Model file for the job. Use its own axes, mm. Face numbers are marked on the shaded views. A direction names the side the tool comes from. Coordinates: 2 decimals unless noted, no trailing zeros. Loops run counter-clockwise (first coordinate to the right, second up) from the corner with the lowest first, then second, coordinate; pieces in that order, holes last.
Autodesk Fusion 360 part; units mm, degrees
sketch "Sketch1" plane through (0, 0, 0) normal (0, 1, 0) x (1, 0, 0)
  line L0 (41.5, 41.5) -> (-41.5, 41.5)
  line L1 (-41.5, -41.5) -> (41.5, -41.5)
  line L2 (-41.5, 41.5) -> (41.5, -41.5) construction
  line L3 (41.5, 41.5) -> (41.5, 17)
  line L4 (41.5, 17) -> (34.5, 17)
  line L5 (-41.5, 41.5) -> (-41.5, 17)
  line L6 (-41.5, 17) -> (-34.5, 17)
  line L7 (-41.5, -17) -> (-34.5, -17)
  line L8 (41.5, -17) -> (34.5, -17)
  line L9 (-34.5, 17) -> (-34.5, -17)
  line L10 (34.5, 17) -> (34.5, -17)
  line L11 (-41.5, 41.5) -> (-41.5, 17)
  line L12 (-41.5, -17) -> (-41.5, -41.5)
  line L13 (-41.5, -41.5) -> (-41.5, -17)
  line L14 (-41.5, 17) -> (-41.5, 41.5)
  line L15 (41.5, -41.5) -> (41.5, -17)
  line L16 (41.5, 17) -> (41.5, 41.5)
  line L17 (41.5, 41.5) -> (41.5, 17)
  line L18 (41.5, -17) -> (41.5, -41.5)
  line L19 (-34.5, 17) -> (-34.5, 8.6)
  line L20 (-34.5, -17) -> (-34.5, -8.6)
  line L21 (34.5, 17) -> (34.5, 8.6)
  line L22 (34.5, -17) -> (34.5, -8.6)
  line L23 (-41.5, 41.5) -> (-33.655, 41.5)
  line L24 (-33.655, 41.5) -> (-41.5, 41.5)
  line L25 (-41.5, 41.5) -> (-41.5, 33.655)
  circle A0 centre (-33.655, 33.655) radius 1.55
  circle A1 centre (33.655, 33.655) radius 1.55
  circle A2 centre (-33.655, -33.655) radius 1.55
  circle A3 centre (33.655, -33.655) radius 1.55
  line L26 (11, 11) -> (-11, -11) construction
  line L27 (-11, 11) -> (11, -11) construction
  line L28 (12.5, -12.5) -> (-12.5, -12.5)
  line L29 (-12.5, -12.5) -> (-12.5, 12.5)
  line L30 (-12.5, 12.5) -> (12.5, 12.5)
  line L31 (12.5, 12.5) -> (12.5, -12.5)
  line L32 (12.5, -12.5) -> (-12.5, 12.5) construction
  line L33 (-12.5, -12.5) -> (12.5, 12.5) construction
  line L34 (-41.5, 41.5) -> (-14.05, 41.5)
  line L35 (-14.05, 41.5) -> (-8.5, 41.5)
  circle A4 centre (-8.5, 33.655) radius 1.55
  circle A5 centre (8.5, 33.655) radius 1.55
  line L36 (-14.05, 41.5) -> (-14.05, 23.5)
  line L37 (-14.05, 23.5) -> (14.05, 23.5)
  line L38 (14.05, 23.5) -> (14.05, 41.5)
  line L39 (-14.05, -23.5) -> (14.05, -23.5)
  circle A6 centre (8.5, -33.655) radius 1.55
  circle A7 centre (-8.5, -33.655) radius 1.55
  line L40 (-14.05, -41.5) -> (-14.05, -23.5)
  line L41 (14.05, -23.5) -> (14.05, -41.5)
  circle A8 centre (-19.5, 8.6) radius 1.55
  circle A9 centre (-19.5, -8.6) radius 1.55
  circle A10 centre (19.5, 8.6) radius 1.55
  circle A11 centre (19.5, -8.6) radius 1.55
  point P0 (-19.5, 8.6)
  point P1 (19.5, 8.6)
  dimension "d1" = 83
  dimension "d2" = 83
  dimension "d31" = 27.45
  dimension "d32" = 5.55
  dimension "d33" = 7.845
  dimension "d34" = 17
  dimension "d35" = 3.1
  dimension "d36" = 3.1
  dimension "d37" = 18
  dimension "d39" = 18
  dimension "d40" = 3.1
extrude "Extrude4" add sketch "Sketch1" along normal blind 8 contours L0 L1 L3 L4 L5 L6 L7 L8 L9 L10 L11 L12 L13 L14 L15 L16 L17 L18 L19 L20 L21 L22 L23 L24 L25 L34 L36 L37 L38 L39 L40 L41 makes body 1
sketch "Sketch2" plane through (0, 8, 0) normal (0, 1, 0) x (-1, 0, 0)
  circle A0 centre (-19.5, -8.6) radius 1.55
  circle A1 centre (33.655, 33.655) radius 1.55
  circle A2 centre (19.5, -8.6) radius 1.55
  circle A3 centre (19.5, 8.6) radius 1.55
  circle A4 centre (-19.5, 8.6) radius 1.55
  line L0 (12.5, -12.5) -> (-12.5, -12.5)
  line L1 (-12.5, -12.5) -> (-12.5, 12.5)
  line L2 (-12.5, 12.5) -> (12.5, 12.5)
  line L3 (12.5, 12.5) -> (12.5, -12.5)
  circle A5 centre (-33.655, -33.655) radius 1.55
  circle A6 centre (33.655, -33.655) radius 1.55
  circle A7 centre (-33.655, 33.655) radius 1.55
  line L4 (41.5, 41.5) -> (14.05, 41.5)
  line L5 (14.05, 41.5) -> (14.05, 23.5)
  line L6 (14.05, 23.5) -> (-14.05, 23.5)
  line L7 (-14.05, 23.5) -> (-14.05, 41.5)
  line L8 (-14.05, 41.5) -> (-41.5, 41.5)
  line L9 (-41.5, 41.5) -> (-41.5, 17)
  line L10 (-41.5, 17) -> (-34.5, 17)
  line L11 (-34.5, 17) -> (-34.5, -17)
  line L12 (-34.5, -17) -> (-41.5, -17)
  line L13 (-41.5, -17) -> (-41.5, -41.5)
  line L14 (-41.5, -41.5) -> (-14.05, -41.5)
  line L15 (-14.05, -41.5) -> (-14.05, -23.5)
  line L16 (-14.05, -23.5) -> (14.05, -23.5)
  line L17 (14.05, -23.5) -> (14.05, -41.5)
  line L18 (14.05, -41.5) -> (41.5, -41.5)
  line L19 (41.5, -41.5) -> (41.5, -17)
  line L20 (41.5, -17) -> (34.5, -17)
  line L21 (34.5, -17) -> (34.5, 17)
  line L22 (34.5, 17) -> (41.5, 17)
  line L23 (41.5, 17) -> (41.5, 41.5)
extrude "Extrude5" cut sketch "Sketch2" against normal blind 3 keep common part bodies 1
sketch "Sketch3" plane through (0, 0, 23.5) normal (0, 0, 1) x (1, 0, 0)
  line L0 (-14.05, 5) -> (14.05, 5)
  line L1 (14.05, 5) -> (14.05, 8)
  line L2 (14.05, 8) -> (-14.05, 8)
  line L3 (-14.05, 8) -> (-14.05, 5)
  line L4 (-14.05, 8) -> (-14.05, 0)
  line L5 (-14.05, 0) -> (14.05, 0)
  line L6 (14.05, 0) -> (14.05, 8)
  line L7 (14.05, 8) -> (-14.05, 8)
  line L8 (-14.05, 8) -> (-14.05, 0)
  line L9 (-14.05, 0) -> (14.05, 0)
  dimension "d47" = 28.1
extrude "Extrude6" add sketch "Sketch3" against normal blind 3 contours L0 L4 L5 L6 L8 L9 bodies 1
extrude "Extrude7" add sketch "Sketch1" against normal blind 3 separate body contours L1 L39 L40 L41 makes body 2
sketch "Sketch4" plane through (0, 0, 23.5) normal (0, 0, 1) x (1, 0, 0)
  line L0 (14.05, 5) -> (14.05, 8)
  line L1 (14.05, 8) -> (-14.05, 8)
  line L2 (-14.05, 8) -> (-14.05, 5)
  line L3 (-14.05, 5) -> (-14.05, 0)
  line L4 (-14.05, 0) -> (14.05, 0)
  line L5 (14.05, 0) -> (14.05, 5)
  line L6 (-14.05, 0) -> (-14.05, -3)
  line L7 (-14.05, -3) -> (14.05, -3)
  line L8 (-14.05, 0) -> (14.05, 0)
  line L9 (14.05, 0) -> (14.05, -3)
  line L10 (14.05, -3) -> (-14.05, -3)
  line L11 (-14.05, -3) -> (-14.05, 0)
  dimension "d52" = 3
  dimension "d53" = 28.1
extrude "Extrude8" add sketch "Sketch4" against normal blind 3 contours L4 L6 L7 L8 L9 L10 L11 bodies 1 2
sketch "Sketch5" plane through (0, 0, -23.5) normal (0, 0, -1) x (-1, 0, 0)
  line L0 (-14.05, 5) -> (14.05, 5)
  line L1 (14.05, 5) -> (14.05, 8)
  line L2 (14.05, 8) -> (-14.05, 8)
  line L3 (-14.05, 8) -> (-14.05, 5)
  line L4 (-14.05, 5) -> (-14.05, -3)
  line L5 (-14.05, -3) -> (14.05, -3)
  line L6 (14.05, -3) -> (-14.05, -3)
  line L7 (-14.05, -3) -> (-14.05, 5)
  line L8 (-14.05, 5) -> (14.05, 5)
  line L9 (14.05, 5) -> (14.05, -3)
  dimension "d56" = 8
  dimension "d57" = 28.1
extrude "Extrude9" add sketch "Sketch5" against normal blind 3 contours L0 L4 L5 L6 L7 L8 L9 bodies 1
extrude "Extrude10" add sketch "Sketch1" against normal blind 3 contours L0 L35 L36 L37 L38 bodies 1
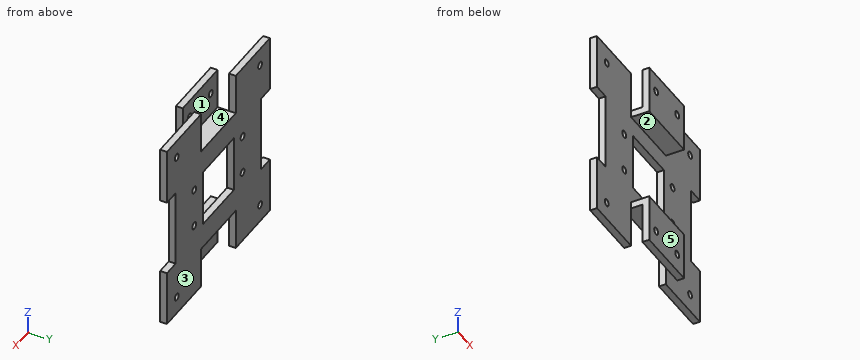
Q1. Slice it at A-A (x = -3). List the corners of the cut face in (y, z).
Answers:
outline: (-3, -41.5) - (0, -41.5) - (0, -23.5) - (8, -23.5) - (8, -12.5) - (5, -12.5) - (5, -20.5) - (-3, -20.5) - close; (-3, 20.5) - (5, 20.5) - (5, 12.5) - (8, 12.5) - (8, 23.5) - (0, 23.5) - (0, 41.5) - (-3, 41.5) - close
Q2. Which spindle directions (+Z, -Z, +X, -X, +Y, -Y) get a long thin tool onto all of the face, cutting with end or side? Do the marked faces 1, 2 and 3. Say none if no direction does.
Answers:
face 1: +Z, +X, -X, +Y
face 2: +X, -X, -Y
face 3: +Z, -Z, +X, -X, +Y
Q3. Slice it at D-D (z = -8.6). List the corners of the cut face in (x, y).
Answers:
outline: (-34.5, 5) - (-21.05, 5) - (-21.05, 8) - (-34.5, 8) - close; (-17.95, 5) - (-12.5, 5) - (-12.5, 8) - (-17.95, 8) - close; (12.5, 5) - (17.95, 5) - (17.95, 8) - (12.5, 8) - close; (21.05, 5) - (34.5, 5) - (34.5, 8) - (21.05, 8) - close
Q4. Slice it at B-B (y = -1.25). List the corners of the cut face in (x, z) (3 decimals).
Answers:
outline: (-14.05, -41.5) - (14.05, -41.5) - (14.05, -20.5) - (-14.05, -20.5) - close; (-14.05, 20.5) - (14.05, 20.5) - (14.05, 41.5) - (-14.05, 41.5) - close; hole circle Ø3.1 at (-8.5, -33.655); hole circle Ø3.1 at (-8.5, 33.655); hole circle Ø3.1 at (8.5, -33.655); hole circle Ø3.1 at (8.5, 33.655)
Q5. Flat gauge pins, fed straight in: P1, Ø0.9, axis at x = -3.5, y = 7, coming from the -Z side; P2, Ø3, axis at x = -8.5, z = 33.655, coming from the +Y side; P3, Ø3.5, axis at y = 6.5, z = -4.5, coming from the -X side; P4, Ø1.5, axis at y = 7, z = 1.5, coming from the +X side. Where does each tip first touch, or does it go through?
Answers:
P1: stops at z = -23.5
P2: passes through
P3: stops at x = -34.5
P4: stops at x = 34.5
Q6. Mould opens along X. For the marked faces 4 and 5 say: +X half, -X half, draft (parallel to the pull), parting line (faces both ways), or undercut.
Answers:
face 4: undercut
face 5: draft
Q7. Slice it at C-C (x = -19.5). List the corners of the cut face in (y, z), and give its area (3 significant figures).
Answers:
outline: (5, -41.5) - (8, -41.5) - (8, -10.15) - (5, -10.15) - close; (5, -7.05) - (8, -7.05) - (8, 7.05) - (5, 7.05) - close; (5, 10.15) - (8, 10.15) - (8, 41.5) - (5, 41.5) - close
area: 230 mm2
Q8. Drill centre lines: line 1 (Z direction, x = -11, y = 1); line 2 (Z direction, x = -19.5, y = 7.3); line 3 (X direction, y = 5.7, z = -8.6). Where is each one in solid material? Low to high.
Answers:
line 1: z = -23.5 to -20.5, 20.5 to 23.5
line 2: z = -41.5 to -10.15, -7.05 to 7.05, 10.15 to 41.5
line 3: x = -34.5 to -21.05, -17.95 to -12.5, 12.5 to 17.95, 21.05 to 34.5
